```python
from build123d import *

# Parameters (mm, degrees)
F0_W     = 139.7
F0_H     = 139.7
F1_DEPTH = 12.7
F2_DEPTH = 12.7


with BuildPart() as f1:
    # F0 (on Top) → F1 (new body)
    with BuildSketch(Plane.XY):
        with BuildLine():
            Line((-206.057255, 215.9), (-206.057255, -215.9))
            ThreePointArc((-206.057255, -215.9), (0, -298.45), (206.057255, -215.9))
            Line((206.057255, -215.9), (206.057255, 215.9))
            Line((206.057255, 215.9), (-206.057255, 215.9))
        make_face()
        with Locations((0, 69.85)):
            Rectangle(F0_W, F0_H, mode=Mode.SUBTRACT)
    extrude(amount=F1_DEPTH)

    # F0 (on Top) → F2 (join)
    with BuildSketch(Plane.XY):
        with BuildLine():
            Line((-206.057255, 215.9), (-206.057255, -215.9))
            ThreePointArc((-206.057255, -215.9), (0, -298.45), (206.057255, -215.9))
            Line((206.057255, -215.9), (206.057255, 215.9))
            Line((206.057255, 215.9), (-206.057255, 215.9))
        make_face()
        with Locations((0, 69.85)):
            Rectangle(F0_W, F0_H, mode=Mode.SUBTRACT)
    extrude(amount=F2_DEPTH)


solid = f1.part
```
For this review, take the finished solid that the model builds, in its own axes (mm). A direction names the side the tool comes from. Give positions to 0.01 mm unless a question says otherwise; leave off trailing zeros. Order: outer loops, then holes, each group sorted by start corner. A loop starts at its lowest first (then second) coordinate and runs counter-clockwise, first axis right, second up.
1) Wall thickness on line 1 (Y direction, x = -0.5, z = 10.25); line 2 (X direction, y = 88, z = 8); line 3 (Y direction, x = 115.5, z = 7.25): over which ranges is each line inside the solid? List them lowest first.
2) Take a section at C-C (x = -47). Give the boundary of the cut face in (y, z), then the cut area to 3 significant figures.
3) For faces 4 (the face through (-1, 139.7, 6)), 5 (the face through (-206.057, 3, 6)), list the 3-axis set-ups (+Z, -Z, +X, -X, +Y, -Y) from which the entire face can be reached by the end or side of a thin tool; tool diameter is ignored.
4) Take a section at D-D (x = -104). Give the boundary of the cut face in (y, z).
5) The part is to be moulded in two halves that separate along Y. For faces 1 (the face through (-3.184, -298.433, 6.261)), 2 (the face through (-1, 0, 6)), 3 (the face through (-3, -38, 0)), say which applies: released by +Y, released by -Y, zero draft, split by the parting line, or undercut.
6) Take a section at A-A (y = 39). Give the boundary of the cut face in (x, z), then the cut area to 3 significant figures.
7) Take a section at B-B (z = 6.5). Give the boundary of the cut face in (x, y).
Derived:
1. line 1: y = -298.45 to 0, 139.7 to 215.9
1. line 2: x = -206.06 to -69.85, 69.85 to 206.06
1. line 3: y = -275.19 to 215.9
2. outline: (-294.73, 0) - (0, 0) - (0, 12.7) - (-294.73, 12.7) - close; (139.7, 0) - (215.9, 0) - (215.9, 12.7) - (139.7, 12.7) - close
2. area: 4,710 mm2
3. face 4: +Z, -Z
3. face 5: +Z, -Z, -X, +Y, -Y
4. outline: (-279.74, 0) - (215.9, 0) - (215.9, 12.7) - (-279.74, 12.7) - close
5. face 1: released by -Y
5. face 2: undercut
5. face 3: zero draft
6. outline: (-206.06, 0) - (-69.85, 0) - (-69.85, 12.7) - (-206.06, 12.7) - close; (69.85, 0) - (206.06, 0) - (206.06, 12.7) - (69.85, 12.7) - close
6. area: 3,460 mm2
7. outline: (-206.06, -215.9) arc R298.45 ccw to (206.06, -215.9) - (206.06, 215.9) - (-206.06, 215.9) - close; hole (-69.85, 0) - (69.85, 0) - (69.85, 139.7) - (-69.85, 139.7) - close
